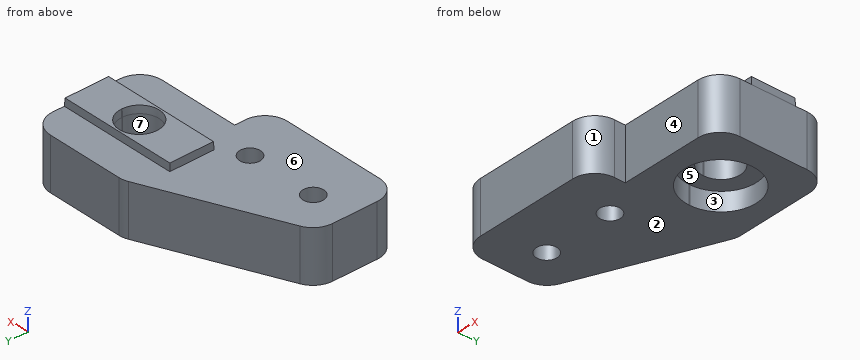
from build123d import *

# Parameters (mm, degrees)
SKETCH1_R           = 1.4
BOSS_EXTRUDE1_DEPTH = 7
CUT_EXTRUDE1_DEPTH  = 2.5
SKETCH3_W           = 16
SKETCH3_H           = 6
BOSS_EXTRUDE2_DEPTH = 1
BOSS_EXTRUDE2_DRAFT = 3


with BuildPart() as part:
    # Sketch1 → Boss-Extrude1 (new body)
    with BuildSketch(Plane.XY):
        with BuildLine():
            Line((3, 0), (17, 0))
            ThreePointArc((17, 0), (19.121320344, 0.878679656), (20, 3))
            Line((20, 3), (20, 4.45))
            Line((20, 4.45), (31, 4.45))
            ThreePointArc((31, 4.45), (33.121320344, 5.328679656), (34, 7.45))
            Line((34, 7.45), (34, 16.55))
            ThreePointArc((34, 16.55), (33.121320344, 18.671320344), (31, 19.55))
            Line((31, 19.55), (20.614357727, 19.55))
            ThreePointArc((20.614357727, 19.55), (20.012490717, 19.489005972), (19.435097237, 19.308504069))
            Line((19.435097237, 19.308504069), (1.820739511, 11.778366141))
            ThreePointArc((1.820739511, 11.778366141), (0.496224704, 10.672468881), (0, 9.019862072))
            Line((0, 9.019862072), (0, 3))
            ThreePointArc((0, 3), (0.878679656, 0.878679656), (3, 0))
        make_face()
        with Locations((5.2, 7)):
            Circle(SKETCH1_R, mode=Mode.SUBTRACT)
        with Locations((14.8, 7)):
            Circle(SKETCH1_R, mode=Mode.SUBTRACT)
        with BuildLine():
            Line((28.6, 12.05), (28.6, 11.95))
            ThreePointArc((28.6, 11.95), (26, 9.35), (23.4, 11.95))
            Line((23.4, 11.95), (23.4, 12.05))
            ThreePointArc((23.4, 12.05), (26, 14.65), (28.6, 12.05))
        make_face(mode=Mode.SUBTRACT)
    extrude(amount=BOSS_EXTRUDE1_DEPTH)

    # Sketch2 → Cut-Extrude1 (cut)
    with BuildSketch(Plane(origin=(0, 0, 0), x_dir=(-1, 0, 0), z_dir=(0, 0, -1))):
        with BuildLine():
            Line((-21.25, 12.05), (-21.25, 11.95))
            ThreePointArc((-21.25, 11.95), (-26, 7.2), (-30.75, 11.95))
            Line((-30.75, 11.95), (-30.75, 12.05))
            ThreePointArc((-30.75, 12.05), (-26, 16.8), (-21.25, 12.05))
        make_face()
    extrude(amount=-CUT_EXTRUDE1_DEPTH, mode=Mode.SUBTRACT)


with BuildPart() as boss_extrude2_tool:
    # Sketch3 → Boss-Extrude2 (with draft: the straight prism first)
    with BuildSketch(Plane.XY.offset(7)):
        with Locations((26, 12)):
            Rectangle(SKETCH3_W, SKETCH3_H)
        with BuildLine():
            Line((28.6, 12.05), (28.6, 11.95))
            ThreePointArc((28.6, 11.95), (26, 9.35), (23.4, 11.95))
            Line((23.4, 11.95), (23.4, 12.05))
            ThreePointArc((23.4, 12.05), (26, 14.65), (28.6, 12.05))
        make_face(mode=Mode.SUBTRACT)
    extrude(amount=BOSS_EXTRUDE2_DEPTH)
    # Boss-Extrude2: the draft: its side faces are tilted about the plane it starts from
    boss_extrude2_sides = [boss_extrude2_tool.faces().sort_by_distance(p)[0] for p in [
        (26, 15, 7.5),
        (18, 12, 7.5),
        (26, 9, 7.5),
        (34, 12, 7.5),
        (26, 14.65, 7.5),
        (28.6, 12, 7.5),
        (26, 9.35, 7.5),
        (23.4, 12, 7.5),
    ]]
    draft(boss_extrude2_sides, Plane.XY.offset(7), BOSS_EXTRUDE2_DRAFT)


with BuildPart() as part_1:
    add(part.part)

    # Boss-Extrude2: add boss_extrude2_tool
    add(boss_extrude2_tool.part)


solid = part_1.part
Can you work these out from the model? Positions are in its coordinate system, mm. Face numbers are marked on the shaded views. A direction names the side the tool comes from. Round coordinates to 2 decimals unless told otherwise and drop trailing zeros. Loops run counter-clockwise (first coordinate to the right, second up) from the corner with the lowest first, then second, coordinate; pieces in that order, holes last. Notation, with made-up numbers: (-28.5, 27.25) - (-0.5, 27.25) arc R25 ccw to (-0.5, 42.25) - close; hole circle Ø9 at (86, 59.25). An arc over 180 degrees is marked (long way). Use CSV: the item, a comma, the result in double quotes. Start each with the question number.
1) If we section it at C-C on x = 14.8: Write out the boundary of the cut face in (y, z).
2) For pin 1 Ø3.5 at (x, z) = (24.5, 3) entering from -Y; pin 2 Ø1.5 at (y, z) = (17, 4) entering from -X; pin 3 Ø3 at (x, z) = (8.5, 7) entering from +Y (3 decimals), each with a flat end and sliding along its axis, tell me the tip position at first contact or that it passes through.
3) If we section it at B-B on x = 26: Write out the boundary of the cut face in (y, z), plus the area to 3 significant figures.
4) We'd pull the mould along X, two halves only. Please class the marked faces 1, 2 and 3: released by +X, released by -X, zero draft, split by the parting line, or undercut.
5) If we section it at D-D on y = 18: Write out the boundary of the cut face in (x, z), plus the area to 3 significant figures.
6) For the marked faces 4, 5, 6 and 7, which set-ups out of +Z, -Z, +X, -X, +Y, -Y let a thin tool reach every point of the face, with its end or its side?
7) If we section it at A-A on z = 4: Write out the boundary of the cut face in (x, y).
8) Please list where these lines run through material, in increasing order: probe 1 along Y at (x, z) = (30, 3); probe 2 along Y at (x, z) = (26, 5.5); probe 3 along Y at (x, z) = (5.2, 3). Write a range as [from, to].
Geometry results:
1,outline,"(0, 0) - (5.6, 0) - (5.6, 7) - (0, 7) - close; (8.4, 0) - (17.33, 0) - (17.33, 7) - (8.4, 7) - close"
2,pin 1,"stops at y = 4.45"
2,pin 2,"stops at x = 12.28"
2,pin 3,"stops at y = 15.275"
3,outline,"(4.45, 0) - (7.2, 0) - (7.2, 2.5) - (9.35, 2.5) - (9.35, 7) - (9.3, 8) - (9.05, 8) - (9, 7) - (4.45, 7) - close; (14.65, 2.5) - (16.8, 2.5) - (16.8, 0) - (19.55, 0) - (19.55, 7) - (15, 7) - (14.95, 8) - (14.7, 8) - (14.65, 7) - close"
3,area,"58.4 mm2"
4,face 1,"released by +X"
4,face 2,"zero draft"
4,face 3,"undercut"
5,outline,"(16.37, 0) - (33.63, 0) - (33.63, 7) - (16.37, 7) - close"
5,area,"121 mm2"
6,face 4,"+Z, -Z, +X, -Y"
6,face 5,"-Z"
6,face 6,"+Z, -X"
6,face 7,"+Z, -Z"
7,outline,"(0, 3) arc R3 ccw to (3, 0) - (17, 0) arc R3 ccw to (20, 3) - (20, 4.45) - (31, 4.45) arc R3 ccw to (34, 7.45) - (34, 16.55) arc R3 ccw to (31, 19.55) - (20.61, 19.55) arc R3 ccw to (19.44, 19.31) - (1.82, 11.78) arc R3 ccw to (0, 9.02) - close; hole circle Ø2.8 at (5.2, 7); hole circle Ø2.8 at (14.8, 7); hole (23.4, 11.95) arc R2.6 ccw to (28.6, 11.95) - (28.6, 12.05) arc R2.6 ccw to (23.4, 12.05) - close"
8,probe 1,"y = [4.45, 19.55]"
8,probe 2,"y = [4.45, 9.35], [14.65, 19.55]"
8,probe 3,"y = [0, 5.6], [8.4, 13.22]"
